For this review, take the finished solid that the model builds, in its own axes (mm). Coordinates: 2 decimals unless noted, no trailing zeros. Order: outer loops, then holes, each group sorted by start corner. A loop starts at its lowest first (then second) coordinate and runs counter-clockwise, first axis right, second up. Notation, with made-up numbers: M -30.5,88 L -6.5,88 A26 cw -6.5,122 Z; hole C -29.5,85.25 d3. An arc over 180 degrees is marked long. Use CSV: the item, a comma, the result in double quotes.
```python
from build123d import *

# Parameters (mm, degrees)
F0_W     = 279.4
F0_H     = 482.6
F1_DEPTH = 25.4


with BuildPart() as f1:
    # F0 (on Front) → F1 (new body)
    with BuildSketch(Plane.XZ):
        Rectangle(F0_W, F0_H)
        Polygon((-95.798433, 110.726304), (-85.160971, 119.429685), (82.137294, 119.429685), (88.906586, 110.726304), align=None, mode=Mode.SUBTRACT)
        Polygon((-93.864352, 141.671643), (-84.19393, 151.342079), (81.170253, 151.342079), (89.873627, 141.671643), align=None, mode=Mode.SUBTRACT)
        Polygon((-93.864352, 169.715866), (-84.19393, 177.452207), (82.137294, 177.452207), (89.873627, 169.715866), align=None, mode=Mode.SUBTRACT)
    extrude(amount=F1_DEPTH)


solid = f1.part
```
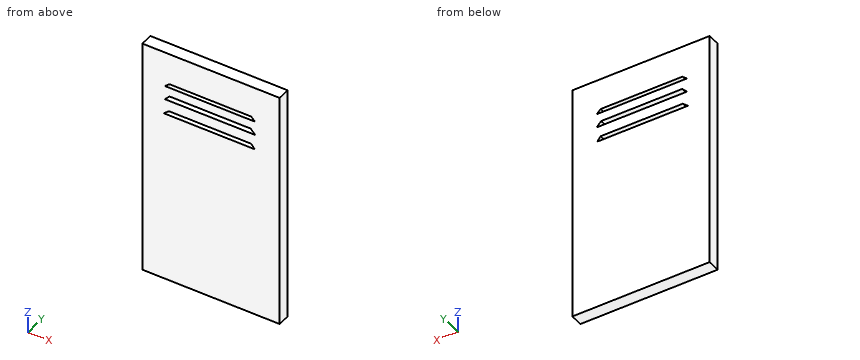
Item 1: Add section B-B on y = -9.25. State the section outline as (x, z) points.
Solutions:
outline,"M -139.7,-241.3 L 139.7,-241.3 L 139.7,241.3 L -139.7,241.3 Z; hole M -95.8,110.73 L 88.91,110.73 L 82.14,119.43 L -85.16,119.43 Z; hole M -93.86,141.67 L 89.87,141.67 L 81.17,151.34 L -84.19,151.34 Z; hole M -93.86,169.72 L 89.87,169.72 L 82.14,177.45 L -84.19,177.45 Z"
Item 2: To check wall thickness, follow line 1 along Z through (x, y) = (12.5, -2.75); line 2 along Z through (x, y) = (85, -3); line 3 along X through (y, z) = (-9.5, 111). State the ranges of each line that lie inside material, in increasing order. Write a range as [from, to].
Solutions:
line 1,"[-241.3, 110.73], [119.43, 141.67], [151.34, 169.72], [177.45, 241.3]"
line 2,"[-241.3, 110.73], [115.75, 141.67], [147.09, 169.72], [174.59, 241.3]"
line 3,"[-139.7, -95.46], [88.69, 139.7]"
Item 3: Add section A-A on x = 34.5. State the section outline as (y, z) points.
Solutions:
outline,"M -25.4,-241.3 L 0,-241.3 L 0,110.73 L -25.4,110.73 Z; M -25.4,119.43 L 0,119.43 L 0,141.67 L -25.4,141.67 Z; M -25.4,151.34 L 0,151.34 L 0,169.72 L -25.4,169.72 Z; M -25.4,177.45 L 0,177.45 L 0,241.3 L -25.4,241.3 Z"
